```python
from build123d import *

# Parameters (mm, degrees)
SKETCH_W        = 61
SKETCH_H        = 30
PAD_DEPTH       = 56
SKETCH003_W     = 40.961635
SKETCH003_H     = 36.049525
POCKET_DEPTH    = 29.8
SKETCH004_W     = 36
SKETCH004_H     = 21
POCKET001_DEPTH = 10
SKETCH005_W     = 26
SKETCH005_H     = 35
POCKET002_DEPTH = 10.1
SKETCH006_W     = 35
SKETCH006_H     = 29.765225
POCKET003_DEPTH = 10.1
SKETCH007_W     = 15
SKETCH007_H     = 33
POCKET004_DEPTH = 10.1
SKETCH009_R     = 2
POCKET005_DEPTH = 5
SKETCH010_R     = 2
POCKET006_DEPTH = 15
SKETCH011_R     = 2
POCKET007_DEPTH = 15
SKETCH012_R     = 2
POCKET008_DEPTH = 15
SKETCH013_W     = 6
SKETCH013_H     = 3
POCKET009_DEPTH = 10
SKETCH014_W     = 6
SKETCH014_H     = 3
POCKET010_DEPTH = 10
SKETCH015_W     = 6
SKETCH015_H     = 3
POCKET011_DEPTH = 10
SKETCH016_W     = 6
SKETCH016_H     = 3
POCKET012_DEPTH = 10


with BuildPart() as part:
    # Sketch → Pad (new body)
    with BuildSketch(Plane.XZ):
        with Locations((9.874064, -12.009427)):
            Rectangle(SKETCH_W, SKETCH_H)
    extrude(amount=PAD_DEPTH)

    # Sketch003 → Pocket (cut)
    with BuildSketch(Plane(origin=(0, 0, -27.009427), x_dir=(1, 0, 0), z_dir=(0, 0, -1))):
        with Locations((9.892656, 28.067419)):
            Rectangle(SKETCH003_W, SKETCH003_H)
    extrude(amount=-POCKET_DEPTH, mode=Mode.SUBTRACT)

    # Sketch004 → Pocket001 (cut)
    with BuildSketch(Plane.XZ.offset(56)):
        with Locations((9.508816, -16.629091)):
            Rectangle(SKETCH004_W, SKETCH004_H)
    extrude(amount=-POCKET001_DEPTH, mode=Mode.SUBTRACT)

    # Sketch005 → Pocket002 (cut)
    with BuildSketch(Plane(origin=(40.374064, 0, 0), x_dir=(0, 0, 1), z_dir=(1, 0, 0))):
        with Locations((-14.2042, 26.235572)):
            Rectangle(SKETCH005_W, SKETCH005_H)
    extrude(amount=-POCKET002_DEPTH, mode=Mode.SUBTRACT)

    # Sketch006 → Pocket003 (cut)
    with BuildSketch(Plane(origin=(0, 0, 0), x_dir=(1, 0, 0), z_dir=(0, 1, 0))):
        with Locations((10.843993, 12.155679)):
            Rectangle(SKETCH006_W, SKETCH006_H)
    extrude(amount=-POCKET003_DEPTH, mode=Mode.SUBTRACT)

    # Sketch007 → Pocket004 (cut)
    with BuildSketch(Plane(origin=(-20.625936, 0, 0), x_dir=(0, 0, -1), z_dir=(-1, 0, 0))):
        with Locations((19.549922, 27.327213)):
            Rectangle(SKETCH007_W, SKETCH007_H)
    extrude(amount=-POCKET004_DEPTH, mode=Mode.SUBTRACT)

    # Sketch009 → Pocket005 (cut)
    with BuildSketch(Plane(origin=(0, 0, -27.009427), x_dir=(1, 0, 0), z_dir=(0, 0, -1))):
        with Locations((-15.002267, 51.059483)):
            Circle(SKETCH009_R)
    extrude(amount=-POCKET005_DEPTH, mode=Mode.SUBTRACT)

    # Sketch010 → Pocket006 (cut)
    with BuildSketch(Plane(origin=(0, 0, -27.009427), x_dir=(1, 0, 0), z_dir=(0, 0, -1))):
        with Locations((35.071098, 50.12505)):
            Circle(SKETCH010_R)
    extrude(amount=-POCKET006_DEPTH, mode=Mode.SUBTRACT)

    # Sketch011 → Pocket007 (cut)
    with BuildSketch(Plane(origin=(0, 0, -27.009427), x_dir=(1, 0, 0), z_dir=(0, 0, -1))):
        with Locations((-15.214926, 4.978576)):
            Circle(SKETCH011_R)
    extrude(amount=-POCKET007_DEPTH, mode=Mode.SUBTRACT)

    # Sketch012 → Pocket008 (cut)
    with BuildSketch(Plane(origin=(0, 0, -27.009427), x_dir=(1, 0, 0), z_dir=(0, 0, -1))):
        with Locations((35.045578, 5.033976)):
            Circle(SKETCH012_R)
    extrude(amount=-POCKET008_DEPTH, mode=Mode.SUBTRACT)

    # Sketch013 → Pocket009 (cut)
    with BuildSketch(Plane.XZ.offset(56)):
        with Locations((34.876442, -21.54185)):
            Rectangle(SKETCH013_W, SKETCH013_H)
    extrude(amount=-POCKET009_DEPTH, mode=Mode.SUBTRACT)

    # Sketch014 → Pocket010 (cut)
    with BuildSketch(Plane.XZ.offset(56)):
        with Locations((-15.041702, -21.455929)):
            Rectangle(SKETCH014_W, SKETCH014_H)
    extrude(amount=-POCKET010_DEPTH, mode=Mode.SUBTRACT)

    # Sketch015 → Pocket011 (cut)
    with BuildSketch(Plane(origin=(0, 0, 0), x_dir=(1, 0, 0), z_dir=(0, 1, 0))):
        with Locations((-15.06067, 21.44039)):
            Rectangle(SKETCH015_W, SKETCH015_H)
    extrude(amount=-POCKET011_DEPTH, mode=Mode.SUBTRACT)

    # Sketch016 → Pocket012 (cut)
    with BuildSketch(Plane(origin=(0, 0, 0), x_dir=(1, 0, 0), z_dir=(0, 1, 0))):
        with Locations((34.804899, 21.419892)):
            Rectangle(SKETCH016_W, SKETCH016_H)
    extrude(amount=-POCKET012_DEPTH, mode=Mode.SUBTRACT)


solid = part.part
```
The listing builds one solid part. Answer for the finished solid, in the listing's coordinates (mm). A direction names the side the tool comes from. Coordinates: 2 decimals unless noted, no trailing zeros. Loops run counter-clockwise (first coordinate to the right, second up) from the corner with the lowest first, then second, coordinate; pieces in that order, holes last. Notation, with made-up numbers: M 40,27 L 63,27 A31 ccw 63,57 Z; hole C 48.25,78.5 d11. An arc over 180 degrees is marked long. Answer as a JSON object with one key per item and string values. Group by question number.
Item 1: Which of the six approach directions +Z, -Z, +X, -X, +Y, -Y give full straight-line access (tool end or side, diameter ignored) to faces 1 (the face through (10, -28, 2.791)), 2 (the face through (35, -26, -1.204)), 3 (the face through (-12.042, -51, -21)), 4 (the face through (-18.061, -5, -21))?
Item 2: Each of these flat-tipped pins is pushed along its axis until it touches: P1, Ø11, axis at x = 3, y = -29.5, coming from the -Z side; P2, Ø12, axis at x = 20.5, z = -0.5, coming from the +Y side; P3, Ø11, axis at x = -17.5, y = -35.5, coming from the -Z side; P4, Ø3, axis at x = 22.5, z = -6.5, coming from the +Y side. Where does it stop, or does it pass through?
Item 3: Section D-D (z = -19) is taken. Write down the section's boundary in (x, y), and give its area (3 significant figures).
Item 4: Consider L1, parallel to Y at x = 38.5, z = -18.5; L2, parallel to Y at x = -13.5, z = -23.5; L3, parallel to X at y = -6.5, z = 0.75. Determine where each line is inside the solid, lowest interval first.
Item 5: Determine the mould class of faces 5 (the face through (35, -46, -22)), 6 (the face through (-16, -43.827, -19)), 7 (the face through (-15, -48, -27.009)), 8 (the face through (-11, 0, -12)) for opening direction Y: +Y half, -Y half, draft (parallel to the pull), parting line (faces both ways), or undercut.
Item 6: Section A-A (z = -10.25) is taken. Write down the section's boundary in (x, y).
Item 7: Section C-C (y = -45) is taken. Write down the section's boundary in (x, z), and give its area (3 significant figures).
Item 8: Section B-B (x = 16.5) is taken. Write down the section's boundary in (y, z).
Solved:
{
 "1": {"face 1": "-Z", "face 2": "-Z, +X", "face 3": "-Y", "face 4": "+Y"},
 "2": {"P1": "stops at z = 2.79", "P2": "stops at y = 0", "P3": "stops at z = -12.05", "P4": "stops at y = -46.09"},
 "3": {"outline": "M -20.63,-56 L -8.49,-56 L -8.49,-46.09 L -10.59,-46.09 L -10.59,-43.83 L -20.63,-43.83 Z; M -20.63,-10.83 L -10.59,-10.83 L -10.59,-10.04 L -6.66,-10.04 L -6.66,0 L -20.63,0 Z; M 27.51,-56 L 40.37,-56 L 40.37,-43.74 L 30.37,-43.74 L 30.37,-46.09 L 27.51,-46.09 Z; M 28.34,-10.04 L 30.27,-10.04 L 30.27,-8.74 L 40.37,-8.74 L 40.37,0 L 28.34,0 Z; hole C -15.21,-4.98 d4; hole C 35.05,-5.03 d4; hole C 35.07,-50.13 d4", "area": "512 mm2"},
 "4": {"L1": "y = -56 to -43.74, -8.74 to 0", "L2": "y = -56 to -52.38, -49.74 to -43.83, -10.83 to -6.01, -3.95 to 0", "L3": "x = -20.63 to -6.66, 28.34 to 40.37"},
 "5": {"face 5": "-Y half", "face 6": "undercut", "face 7": "draft", "face 8": "+Y half"},
 "6": {"outline": "M -20.63,-56 L -8.49,-56 L -8.49,-46.09 L -10.59,-46.09 L -10.59,-10.04 L -6.66,-10.04 L -6.66,0 L -20.63,0 Z; M 27.51,-56 L 40.37,-56 L 40.37,-43.74 L 30.37,-43.74 L 30.37,-46.09 L 27.51,-46.09 Z; M 28.34,-10.04 L 30.27,-10.04 L 30.27,-8.74 L 40.37,-8.74 L 40.37,0 L 28.34,0 Z"},
 "7": {"outline": "M -20.63,-27.01 L -10.59,-27.01 L -10.59,2.79 L 30.37,2.79 L 30.37,-27.01 L 40.37,-27.01 L 40.37,2.99 L -20.63,2.99 Z", "area": "609 mm2"},
 "8": {"outline": "M -56,-6.13 L -46.09,-6.13 L -46.09,2.79 L -10.04,2.79 L -10.04,2.73 L 0,2.73 L 0,2.99 L -56,2.99 Z"}
}
